Could you check a few things on this model? Use its own coordinates, in mm. Face numbers are marked on the shaded views. Round coordinates to 2 decimals unless told otherwise and drop trailing zeros. Loops run counter-clockwise (first coordinate to the right, second up) from the corner with the lowest first, then second, coordinate; pieces in that order, holes last. Notation, with made-up numbers: (-25, 52.5) - (-3, 52.5) arc R31 cw to (-3, 89.5) - close; hole circle Ø5 at (-0.5, 14). An arc over 180 degrees is marked (long way). Answer as CSV lines item,"result". Start each with the question number.
1) I'm going to push flat-ended pins straight in: pin 1 Ø4.5 at (y, z) = (1.5, 1.5) entering from +X; pin 2 Ø1.5 at (x, z) = (5, -3) entering from +Y; pin 3 Ø1.5 at (x, z) = (-11.5, -6) entering from -Y; pin 4 Ø5 at (x, y) = (10, -3) entering from -Z. Where does each tip first touch, or does it pass through?
2) Suppose I cut it at A-A, the plane x = -4. Write out the boundary of the cut face in (y, z), then the cut area to 3 significant figures.
3) We'd pull the mould along Y, two halves only. Please class the marked faces 1, 2 and 3: pulls with the +Y half, pulls with the -Y half, needs draft (parallel to the pull), parting line crosses it, or undercut.
4) Please list where these lines run through material, in increasing order: line 1 along X through (y, z) = (-3, -2); line 2 along Z through (x, y) = (-16.5, -0.25); line 3 along Y through (x, z) = (8, -28).
5) Suppose I cut it at B-B, the plane y = -1. Write out the boundary of the cut face in (x, z).
6) Suppose I cut it at D-D, the plane x = -10. Write out the boundary of the cut face in (y, z), then the cut area to 3 significant figures.
7) Suppose I cut it at C-C, the plane z = -17. Write out the boundary of the cut face in (x, y), then the cut area to 3 significant figures.
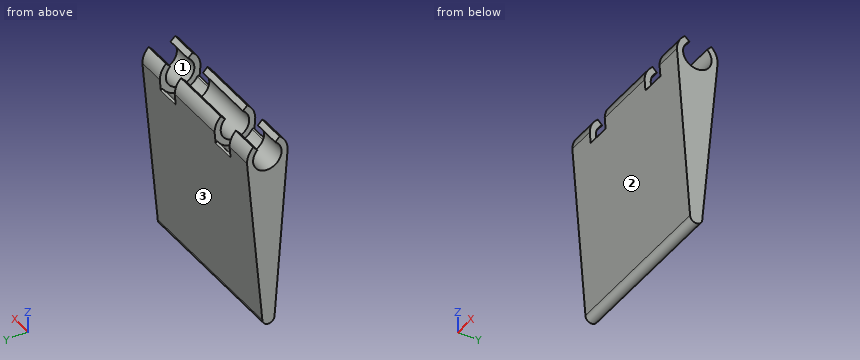
```python
from build123d import *

# Parameters (mm, degrees)
SKETCH1_R           = 3.5
SKETCH1_R_2         = 1.500000000000004
BOSS_EXTRUDE1_DEPTH = 21
CUT_EXTRUDE1_START  = 14
SKETCH1_3_R         = 3.5
CUT_EXTRUDE1_DEPTH  = 6
CUT_EXTRUDE2_START  = -8
SKETCH1_4_R         = 3.5
CUT_EXTRUDE2_DEPTH  = 6
FILLET2_R           = 0.3
CUT_EXTRUDE3_REACH  = 62.673


with BuildPart() as part:
    # Sketch1 → Boss-Extrude1 (new, symmetric)
    # profile 1 of 3: a face of its own
    with BuildSketch(Plane(origin=(0, 0, 0), x_dir=(0, 0, -1), z_dir=(1, 0, 0))):
        with BuildLine():
            ThreePointArc((42, -1.7814888188261242), (40.49999999999999, -0.2814888188261199), (42, 1.2185111811738838))
            Line((42, 1.21851118117388), (0.8931145530180302, 4.919588031043605))
            ThreePointArc((0.8931145530180298, 4.919588031043595), (3.8383311976098513, 3.204249306382842), (5, 0))
            ThreePointArc((5, -1.22e-15), (3.7953387230389426, -3.255058214133985), (0.7618384090395492, -4.9416193943394795))
            Line((0.7618384090395499, -4.9416193943394875), (42, -1.7814888188261202))
        make_face()
    # profile 2 of 3: a face of its own
    with BuildSketch(Plane(origin=(0, 0, 0), x_dir=(0, 0, -1), z_dir=(1, 0, 0))):
        with BuildLine():
            ThreePointArc((5, 0), (3.8383311976098513, 3.204249306382842), (0.8931145530180298, 4.919588031043595))
            Line((0.8931145530180302, 4.919588031043605), (0, 5))
            ThreePointArc((3.1e-16, 5), (-5, 6.1e-16), (-9.2e-16, -5))
            Line((0, -5), (0.7618384090395499, -4.9416193943394875))
            ThreePointArc((0.7618384090395492, -4.9416193943394795), (3.7953387230389426, -3.255058214133985), (5, -1.22e-15))
        make_face()
        with Locations(Location((0, 0, 0), (0, 0, 180))):
            Circle(SKETCH1_R, mode=Mode.SUBTRACT)
    # profile 3 of 3: a face of its own
    with BuildSketch(Plane(origin=(0, 0, 0), x_dir=(0, 0, -1), z_dir=(1, 0, 0))):
        with Locations((42, -0.2814888188261201)):
            Circle(SKETCH1_R_2)
    extrude(amount=BOSS_EXTRUDE1_DEPTH, both=True)

    # Sketch1<3> → Cut-Extrude1 (cut)
    with BuildSketch(Plane(origin=(0, 0, 0), x_dir=(0, 0, -1), z_dir=(1, 0, 0)).offset(CUT_EXTRUDE1_START)):
        with BuildLine():
            ThreePointArc((5, 0), (3.8383311976098513, 3.204249306382842), (0.8931145530180298, 4.919588031043595))
            Line((0.8931145530180302, 4.919588031043605), (0, 5))
            ThreePointArc((3.1e-16, 5), (-5, 6.1e-16), (-9.2e-16, -5))
            Line((0, -5), (0.7618384090395499, -4.9416193943394875))
            ThreePointArc((0.7618384090395492, -4.9416193943394795), (3.7953387230389426, -3.255058214133985), (5, -1.22e-15))
        make_face()
        with Locations(Location((0, 0, 0), (0, 0, 180))):
            Circle(SKETCH1_3_R, mode=Mode.SUBTRACT)
    extrude(amount=-CUT_EXTRUDE1_DEPTH, mode=Mode.SUBTRACT)

    # Sketch1<4> → Cut-Extrude2 (cut)
    with BuildSketch(Plane(origin=(0, 0, 0), x_dir=(0, 0, -1), z_dir=(1, 0, 0)).offset(CUT_EXTRUDE2_START)):
        with BuildLine():
            ThreePointArc((5, 0), (3.8383311976098513, 3.204249306382842), (0.8931145530180298, 4.919588031043595))
            Line((0.8931145530180302, 4.919588031043605), (0, 5))
            ThreePointArc((3.1e-16, 5), (-5, 6.1e-16), (-9.2e-16, -5))
            Line((0, -5), (0.7618384090395499, -4.9416193943394875))
            ThreePointArc((0.7618384090395492, -4.9416193943394795), (3.7953387230389426, -3.255058214133985), (5, -1.22e-15))
        make_face()
        with Locations(Location((0, 0, 0), (0, 0, 180))):
            Circle(SKETCH1_4_R, mode=Mode.SUBTRACT)
    extrude(amount=-CUT_EXTRUDE2_DEPTH, mode=Mode.SUBTRACT)

    # Fillet2
    fillet2_edges = [part.edges().sort_by_distance(p)[0] for p in [
        (11, 4.919588031043601, -0.8931145530180298),
        (11, -4.941619394339483, -0.7618384090395496),
        (-11, 4.919588031043601, -0.8931145530180298),
        (-11, -4.941619394339483, -0.7618384090395496),
    ]]
    fillet(fillet2_edges, radius=FILLET2_R)

    # Cut-Extrude3: up to this face of the body (flat: up to its plane)
    cut_extrude3_end = Plane(part.part.faces().sort_by_distance((-21, -0.117271195, -17.205258384))[0])
    # Sketch2 → Cut-Extrude3 (cut, up to the picked face)
    with BuildSketch(Plane(origin=(21, 0, 0), x_dir=(0, 0, -1), z_dir=(1, 0, 0)), mode=Mode.PRIVATE) as cut_extrude3_sk1:
        with BuildLine():
            Line((-3.6020994823407393, 3.467690776196831), (-2.5214696376385177, 2.4273835433377813))
            ThreePointArc((-2.5214696376385177, 2.4273835433377813), (-3.486645137099691, 0.30545979758239905), (-2.905137986458371, -1.9519665160131723))
            Line((-2.905137986458371, -1.9519665160131723), (-3.979850788994912, -3.026679318549717))
            ThreePointArc((-3.979850788994912, -3.026679318549717), (-4.991563203159533, 0.2903390928961196), (-3.6020994823407393, 3.467690776196831))
        make_face()
    cut_extrude3_tool1 = split(extrude(cut_extrude3_sk1.sketch, amount=-CUT_EXTRUDE3_REACH, mode=Mode.PRIVATE), bisect_by=cut_extrude3_end, keep=Keep.BOTH, mode=Mode.PRIVATE)
    add(cut_extrude3_tool1.solids().sort_by(Axis((21, 0.27388, 3.94965), (-1, 0, 0)))[0], mode=Mode.SUBTRACT)


solid = part.part
```
Filled sheet:
1,pin 1,"x = 21"
1,pin 2,"y = 4.8"
1,pin 3,"y = -4.6"
1,pin 4,"z = -43.48"
2,outline,"(-5, 0) - (-1.78, -42) arc R1.5 ccw to (1.22, -42) - (5, 0) arc R5 ccw to (3.47, 3.6) - (2.43, 2.52) arc R3.5 cw (long way) to (-1.95, 2.91) - (-3.03, 3.98) arc R5 ccw to start"
2,area,"268 mm²"
3,face 1,"undercut"
3,face 2,"pulls with the -Y half"
3,face 3,"pulls with the +Y half"
4,line 1,"-21 to -14, -8 to 8, 14 to 21"
4,line 2,"-43.5 to -3.49"
4,line 3,"-2.85 to 2.48"
5,outline,"(-21, -43.32) - (21, -43.32) - (21, -3.35) - (14, -3.35) - (14, -4.9) - (8, -4.9) - (8, -3.35) - (-8, -3.35) - (-8, -4.9) - (-14, -4.9) - (-14, -3.35) - (-21, -3.35) - close"
6,outline,"(-4.78, -2.85) - (-1.78, -42) arc R1.5 ccw to (1.22, -42) - (4.74, -2.92) arc R0.3 ccw to (4.19, -2.73) arc R5 cw to (-4.23, -2.67) arc R0.3 ccw to start"
6,area,"237 mm²"
7,outline,"(-21, -3.7) - (21, -3.7) - (21, 3.47) - (-21, 3.47) - close"
7,area,"301 mm²"
